Solid Edge part; units mm, degrees
sketch "Sketch1" plane through (0, 0, 0) normal (0, 0, 1) x (1, 0, 0)
  line L0 (0, 0) -> (60, 0)
  line L1 (60, 0) -> (60, 30)
  line L2 (60, 30) -> (0, 30)
  line L3 (0, 30) -> (0, 0)
extrude "Protrusion1" add sketch "Sketch1" along normal blind 2
sketch "Sketch2" plane through (0, 0, 0) normal (1, 0, 0) x (0, 1, 0)
  circle A0 centre (0, 1) radius 5
extrude "拉伸_2" add sketch "Sketch2" along normal blind 15
sketch "Sketch3" plane through (45, 0, 0) normal (1, 0, 0) x (0, 1, 0)
  circle A0 centre (0, 1) radius 5
extrude "拉伸_3" add sketch "Sketch3" along normal blind 15
sketch "Sketch4" plane through (0, 0, 0) normal (1, 0, 0) x (0, 1, 0)
  circle A0 centre (0, 1) radius 3.2
extrude "拉伸除料_1" cut sketch "Sketch4" along normal blind 15
sketch "Sketch5" plane through (45, 0, 0) normal (1, 0, 0) x (0, 1, 0)
  circle A0 centre (0, 1) radius 3.2
extrude "拉伸除料_2" cut sketch "Sketch5" along normal blind 15
Verification items for the finished model (mm, model axes). A direction names the side the tool comes from. Give positions to 0.01 mm unless a question says otherwise; leave off trailing zeros. Order: outer loops, then holes, each group sorted by start corner. A loop starts at its lowest first (then second) coordinate and runs counter-clockwise, first axis right, second up. Notation, with made-up numbers: M -11,68 L 40,68 A13 ccw 40,89 Z; hole C 16.25,85.5 d11. An arc over 180 degrees is marked long. Answer as a JSON object with one key per item and string values. Group by question number.
1) Depth check by flat-ended pin: pin 1 Ø4 at (y, z) = (0, 1) entering from +X; pin 2 Ø1 at (y, z) = (1.5, 0.5) entering from -X; pin 3 Ø1 at (x, z) = (25.5, 1) entering from -Y. Enter the tip coordinate at first touch or a pass-through.
2) Scan lines: line 1 along Y through (x, z) = (49.5, 1); line 2 along Z through (x, y) = (8, 0); line 3 along Z through (x, y) = (13.5, 25.5). Record each from-to range of solid material in increasing order. Write a range as [from, to].
3) Cross-section at C-C (x = 9.5). Enter the section's corners in (y, z), then the cut area to 3 significant figures.
4) Cross-section at A-A (z = 1). Enter the section's corners in (x, y).
5) Mould release check, pull along Y, two halves, no side actions. Record for faces 1 (the face through (7, -5, 1)), 2 (the face through (0, 9, 1)), 3 (the face through (45, 2, 1)): released by +Y, released by -Y, zero draft, split by the parting line, or undercut.
6) Access from +Z, -Z, +X, -X, +Y, -Y to the whole of each face (thin tool, end or side, straight path). Record for faces 4 (the face through (30, 30, 1)), 5 (the face through (15, 2, 1)).
7) Cross-section at B-B (y = -1). Enter the section's corners in (x, z), then the cut area to 3 significant figures.
8) Cross-section at D-D (x = 33). Enter the section's corners in (y, z), then the cut area to 3 significant figures.
Result sheet:
{
 "1": {"pin 1": "stops at x = 45", "pin 2": "stops at x = 15", "pin 3": "stops at y = 0"},
 "2": {"line 1": "y = [-5, -3.2], [3.2, 30]", "line 2": "z = [-4, -2.2], [4.2, 6]", "line 3": "z = [0, 2]"},
 "3": {"outline": "M 4.9,0 L 30,0 L 30,2 L 4.9,2 A5 ccw long Z; hole C 0,1 d6.4", "area": "96.4 mm2"},
 "4": {"outline": "M 0,-5 L 15,-5 L 15,-3.2 L 0,-3.2 Z; M 0,3.2 L 15,3.2 L 15,0 L 45,0 L 45,3.2 L 60,3.2 L 60,30 L 0,30 Z; M 45,-5 L 60,-5 L 60,-3.2 L 45,-3.2 Z"},
 "5": {"face 1": "split by the parting line", "face 2": "zero draft", "face 3": "undercut"},
 "6": {"face 4": "+Z, -Z, +X, -X, +Y", "face 5": "-X"},
 "7": {"outline": "M 0,-3.9 L 15,-3.9 L 15,-2.04 L 0,-2.04 Z; M 0,4.04 L 15,4.04 L 15,5.9 L 0,5.9 Z; M 45,-3.9 L 60,-3.9 L 60,-2.04 L 45,-2.04 Z; M 45,4.04 L 60,4.04 L 60,5.9 L 45,5.9 Z", "area": "112 mm2"},
 "8": {"outline": "M 0,0 L 30,0 L 30,2 L 0,2 Z", "area": "60.0 mm2"}
}
